from build123d import *

# Parameters (mm, degrees)
SKETCH1_W           = 35
SKETCH1_H           = 20
SKETCH1_W_2         = 32
SKETCH1_H_2         = 17
BOSS_EXTRUDE1_DEPTH = 5
SKETCH2_W           = 32
SKETCH2_H           = 17
BOSS_EXTRUDE2_DEPTH = 1.5
SKETCH3_R           = 2.4
BOSS_EXTRUDE3_DEPTH = 1.8
SKETCH6_R           = 3.25
SKETCH6_R_2         = 2.4
BOSS_EXTRUDE4_DEPTH = 3.5
SKETCH7_R           = 0.9
CUT_EXTRUDE2_DEPTH  = 1.8


with BuildPart() as part:
    # Sketch1 → Boss-Extrude1 (new body)
    with BuildSketch(Plane.XY):
        Rectangle(SKETCH1_W, SKETCH1_H)
        Rectangle(SKETCH1_W_2, SKETCH1_H_2, mode=Mode.SUBTRACT)
    extrude(amount=BOSS_EXTRUDE1_DEPTH)

    # Sketch2 → Boss-Extrude2 (add)
    with BuildSketch(Plane.XY):
        Rectangle(SKETCH2_W, SKETCH2_H)
    extrude(amount=BOSS_EXTRUDE2_DEPTH)

    # Sketch3 → Boss-Extrude3 (add)
    with BuildSketch(Plane(origin=(0, 0, 0), x_dir=(-1, 0, 0), z_dir=(0, 0, -1))):
        with BuildLine():
            ThreePointArc((15.15, -5), (14.447056275, -3.302943725), (12.75, -2.6))
            Line((12.75, -2.6), (12.75, -5))
            Line((12.75, -5), (15.15, -5))
        make_face()
        with BuildLine():
            Line((12.75, -5), (12.75, -2.6))
            ThreePointArc((12.75, -2.6), (11.052943725, -3.302943725), (10.35, -5))
            Line((10.35, -5), (12.75, -5))
        make_face()
        with BuildLine():
            Line((12.75, -7.4), (12.75, -5))
            Line((12.75, -5), (10.35, -5))
            ThreePointArc((10.35, -5), (11.052943725, -6.697056275), (12.75, -7.4))
        make_face()
        with BuildLine():
            Line((15.15, -5), (12.75, -5))
            Line((12.75, -5), (12.75, -7.4))
            ThreePointArc((12.75, -7.4), (14.447056275, -6.697056275), (15.15, -5))
        make_face()
        with Locations((12.75, 5)):
            Circle(SKETCH3_R)
        with Locations((-4.75, 5)):
            Circle(SKETCH3_R)
        with Locations((-4.75, -5)):
            Circle(SKETCH3_R)
        with Locations((-12.75, -5)):
            Circle(SKETCH3_R)
        with Locations((-12.75, 5)):
            Circle(SKETCH3_R)
        with Locations((4.75, -5)):
            Circle(SKETCH3_R)
        with Locations(Location((4.75, 5, 0), (0, 0, 180))):
            Circle(SKETCH3_R)
    extrude(amount=BOSS_EXTRUDE3_DEPTH)

    # Sketch6 → Boss-Extrude4 (add)
    # profile 1 of 3: a face of its own
    with BuildSketch(Plane.XY.offset(1.5)):
        Circle(SKETCH6_R)
        Circle(SKETCH6_R_2, mode=Mode.SUBTRACT)
    # profile 2 of 3: a face of its own
    with BuildSketch(Plane.XY.offset(1.5)):
        with Locations((8, 0)):
            Circle(SKETCH6_R)
        with Locations((8, 0)):
            Circle(SKETCH6_R_2, mode=Mode.SUBTRACT)
    # profile 3 of 3: a face of its own
    with BuildSketch(Plane.XY.offset(1.5)):
        with Locations(Location((-8, 0, 0), (0, 0, 180))):
            Circle(SKETCH6_R)
        with Locations(Location((-8, 0, 0), (0, 0, 180))):
            Circle(SKETCH6_R_2, mode=Mode.SUBTRACT)
    extrude(amount=BOSS_EXTRUDE4_DEPTH)

    # Sketch7 → Cut-Extrude2 (cut)
    with BuildSketch(Plane.XY.offset(1.5)):
        with Locations((12.75, 5)):
            Circle(SKETCH7_R)
        with Locations((-12.75, 5)):
            Circle(SKETCH7_R)
        with Locations((-12.75, -5)):
            Circle(SKETCH7_R)
        with Locations((-4.75, -5)):
            Circle(SKETCH7_R)
        with Locations((12.75, -5)):
            Circle(SKETCH7_R)
        with Locations(Location((4.75, 5, 0), (0, 0, 180))):
            Circle(SKETCH7_R)
        with Locations((-4.75, 5)):
            Circle(SKETCH7_R)
        with Locations((4.75, -5)):
            Circle(SKETCH7_R)
    extrude(amount=-CUT_EXTRUDE2_DEPTH, mode=Mode.SUBTRACT)


solid = part.part
The model under review builds one solid part; all positions refer to its coordinate system, in mm. A direction names the side the tool comes from. Round coordinates to 2 decimals unless told otherwise and drop trailing zeros. Write each loop counter-clockwise with the first axis right and the second up, starting at its lowest first coordinate (ties: lowest second). Pieces come first, ordered by that corner, then holes. Notation, with made-up numbers: M 30.25,29.5 L 52.25,29.5 A18 cw 52.25,63.5 Z; hole C -23.5,-19.75 d2. An arc over 180 degrees is marked long. Answer as CSV lines item,"result". Start each with the question number.
Q1. Wall thickness on line 1 along Y through (x, z) = (8, 4.15); line 2 along Y through (x, z) = (12.75, 0.5); line 3 along Y through (x, z) = (5.5, 4.5): over which ranges is each line inside the solid? List them lowest first.
Q2. Consider section B-B, the plane z = 0.5. State how many separate pieces and enclosed holes the cut face has, then the cut area to 3 significant figures.
Q3. Consider section A-A, the plane z = 2.25. Give the boundary of the cut face in (x, y), then the cut area to 3 significant figures.
Q4. Clearance check with flat-ended pins moving along their axes: P1, Ø0.9, axis at x = -4.5, y = 5, coming from the +Z side; P2, Ø2.5, axis at x = 12.75, y = -5, coming from the +Z side; P3, Ø6, axis at x = 8, y = 0, coming from the -Z side. State where each tip first meets the part, or that it passes through.
Q5. The part is to be moulded in two halves that separate along X. For faces 1 (the face through (0, 10, 2)), 2 (the face through (15.148, -4.894, -0.887)), 3 (the face through (-17.5, 0, 2)), say which applies: +X half, -X half, draft (parallel to the pull), parting line (faces both ways), or undercut.
Q6. Tool access review of faces 4 (the face through (13, 5, -1.8)), 5 (the face through (0, 0, 0)), 6 (the face through (-4, 0, 1.5)): name each direction out of +Z, -Z, +X, -X, +Y, -Y from which nothing blocks a thin tool from reaching the whole face with its end or side.
Q7. Consider section D-D, the plane x = -8. Give the boundary of the cut face in (y, z).
Result set:
1,line 1,"y = -10 to -8.5, -3.25 to -2.4, 2.4 to 3.25, 8.5 to 10"
1,line 2,"y = -10 to -5.9, -4.1 to 4.1, 5.9 to 10"
1,line 3,"y = -10 to -8.5, -2.08 to 2.08, 8.5 to 10"
2,separate pieces,"1"
2,enclosed holes,"8"
2,area,"680 mm²"
3,outline,"M -17.5,-10 L 17.5,-10 L 17.5,10 L -17.5,10 Z; C -8,0 d6.5; C 0,0 d6.5; C 8,0 d6.5; hole M -16,-8.5 L 16,-8.5 L 16,8.5 L -16,8.5 Z; hole C -8,0 d4.8; hole C 0,0 d4.8; hole C 8,0 d4.8"
3,area,"201 mm²"
4,P1,"stops at z = -0.3"
4,P2,"stops at z = 1.5"
4,P3,"stops at z = 0"
5,face 1,"draft"
5,face 2,"undercut"
5,face 3,"-X half"
6,face 4,"-Z, +X, -X, +Y, -Y"
6,face 5,"-Z"
6,face 6,"+Z"
7,outline,"M -10,0 L 10,0 L 10,5 L 8.5,5 L 8.5,1.5 L 3.25,1.5 L 3.25,5 L 2.4,5 L 2.4,1.5 L -2.4,1.5 L -2.4,5 L -3.25,5 L -3.25,1.5 L -8.5,1.5 L -8.5,5 L -10,5 Z"
